Here's how the part is built. I have some questions about the finished solid (model axes, mm). Face numbers are marked on the shaded views. A direction names the side the tool comes from. Coordinates: 2 decimals unless noted, no trailing zeros. Write each loop counter-clockwise with the first axis right and the second up, starting at its lowest first coordinate (ties: lowest second). Pieces come first, ordered by that corner, then holes. Notation, with made-up numbers: (15.5, 24.25) -> (23.5, 24.25) arc R10 ccw to (23.5, 31.25) -> close; hole circle Ø9 at (54, -17). An arc over 180 degrees is marked (long way). Put each result on its own line as item: value. Start each with the question number.
Item 1: On a 3-axis mill with a long thin cutter (end or side, diameter ignored), from which of +Z, -Z, +X, -X, +Y, -Y can I reach the whole of each face in a straight line? I mean the marked faces 5, 6, 7, 8 and 9. Say none if no direction works.
Item 2: I want a section at C-C, the plane z = 15. State how many separate pieces and enclosed holes the cut face has, then the cut area to 3 significant figures.
Item 3: For pin 1 (1.5 mm diameter, centred on x = 102.5, z = 7, fed in from +Y); pin 2 (4 mm diameter, centred on x = 70, z = 23, fed in from -Y); pin 3 (13 mm diameter, centred on x = 114.5, z = 18, fed in from +Y); pin 4 (3 mm diameter, centred on y = -4.5, z = 17, fed in from -X), each with a flat end and sliding along its axis, tell me the tip position at first contact or that it passes through.
Item 4: If we mould it in two halves opening along Z, with no side actions, what happens to the marked faces 1, 2, 3 and 4? For each: released by +Z, released by -Z, zero draft, split by the parting line, or undercut.
Item 5: I want a section at B-B, the plane x = 21.5. List the corners of the cut face in (y, z) for me, then the cut area to 3 significant figures.
Item 6: I need wall thicknesses on line 1 (X direction, y = 16.05, z = 15); line 2 (Z direction, x = 70, y = 15.7); line 3 (Z direction, x = 78, y = 17.8). Which ranges of each line are inside material? Lowest first, please. Write a range as [from, to].
Item 7: I want a section at A-A, the plane y = 10.5. List the corners of the cut face in (x, z) for me.
Autodesk Inventor part; units mm, degrees
ref_plane "YZ Plane" through (0, 0, 0) normal (1, 0, 0) x (0, 1, 0)
ref_plane "XZ Plane" through (0, 0, 0) normal (0, 1, 0) x (-1, 0, 0)
ref_plane "XY Plane" through (0, 0, 0) normal (0, 0, 1) x (1, 0, 0)
sketch "Sketch1" plane through (0, 0, 0) normal (0, 0, 1) x (1, 0, 0)
  line L0 (5, 0) -> (50, 0)
  line L1 (50, 0) -> (50, 18)
  line L2 (52, 20) -> (88, 20)
  line L3 (90, 18) -> (90, 0)
  line L4 (105, 0) -> (135, 0)
  line L5 (140, -5) -> (140, -10)
  line L6 (140, -10) -> (87, -10)
  line L7 (53, -10) -> (0, -10)
  line L8 (0, -10) -> (0, -5)
  line L9 (57, 15) -> (83, 15)
  line L10 (55, 13) -> (55, -8)
  line L11 (85, -8) -> (85, 13)
  arc A0 (52, 20) -> (50, 18) centre (52, 18) ccw
  arc A1 (90, 18) -> (88, 20) centre (88, 18) ccw
  line L12 (50, 9) -> (35, 0)
  line L13 (90, 0) -> (90, 9)
  line L14 (90, 9) -> (105, 0)
  arc A2 (57, 15) -> (55, 13) centre (57, 13) ccw
  arc A3 (85, 13) -> (83, 15) centre (83, 13) ccw
  arc A4 (53, -10) -> (55, -8) centre (53, -8) ccw
  arc A5 (85, -8) -> (87, -10) centre (87, -8) ccw
  line L15 (5, 0) -> (0, -5)
  line L16 (135, 0) -> (140, -5)
  point P0 (0, 0)
  point P1 (50, 20)
  point P2 (90, 20)
  point P3 (140, 0)
  point P4 (140, 0)
  point P5 (0, 0)
  point P6 (140, 0)
  dimension "d0" = 50
  dimension "d1" = 20
  dimension "d2" = 40
  dimension "d3" = 50
  dimension "d4" = 10
  dimension "d7" = 10
  dimension "d8" = 5
  dimension "d9" = 2
  dimension "d10" = 15
  dimension "d11" = 9
  dimension "d12" = 15
  dimension "d13" = 2
  dimension "d14" = 30
  dimension "d15" = 2
  dimension "d18" = 5
  dimension "d19" = 5
  dimension "d20" = 5
  dimension "d21" = 5
extrude "Extrusion1" add sketch "Sketch1" along normal blind 30
sketch "Sketch2" plane through (105, 0, 0) normal (0, 1, 0) x (1, 0, 0)
  circle A0 centre (15, -15) radius 6.5
  line L0 (30, 0) -> (0, 0)
  line L1 (0, 0) -> (0, -30)
  circle A1 centre (-84.9999, -15) radius 6.5
  line L2 (-100, 0) -> (-100, -30)
  line L3 (-70, 0) -> (-100, 0)
  point P0 (-105, 0)
  point P1 (0, -15)
  dimension "d24" = 13
  dimension "d25" = 15
  dimension "d26" = 15
  dimension "d27" = 13
  dimension "d28" = 15
  dimension "d29" = 15
extrude "Extrusion2" cut sketch "Sketch2" against normal blind 30
sketch "Sketch3" plane through (0, 0, 30) normal (0, 0, 1) x (1, 0, 0)
  point P0 (0, 0)
sketch "Sketch4" plane through (52, 20, 0) normal (0, 1, 0) x (1, 0, 0)
  circle A0 centre (18, -15) radius 11.75
  line L0 (38, 0) -> (38, -30)
  line L1 (36, 0) -> (0, 0)
  circle A1 centre (18, -7) radius 1.6
  circle A2 centre (10, -15) radius 1.6
  circle A3 centre (18, -23) radius 1.6
  circle A4 centre (26, -15) radius 1.6
  point P0 (-52, 0)
  dimension "d32" = 23.5
  dimension "d33" = 20
  dimension "d34" = 15
  dimension "d35" = 3.2
  dimension "d36" = 8
  dimension "d39" = 360
extrude "Extrusion3" cut sketch "Sketch4" against normal blind 1.5
extrude "Extrusion4" cut sketch "Sketch4" against normal blind 30 contours A1 | A2 | A3 | A4
fillet "Fillet1" radius 2 18 edges at (50.5858, 19.4142, 0) (50, 13.5, 0) (89.4142, 19.4142, 0) (90, 13.5, 0) (70, 20, 0) (50.5858, 19.4142, 30) (50, 13.5, 30) (89.4142, 19.4142, 30) (90, 13.5, 30) (70, 20, 30) (97.5, 4.5, 30) (120, 0, 30) (97.5, 4.5, 0) (120, 0, 0) (42.5, 4.5, 30) (20, 0, 30) (20, 0, 0) (42.5, 4.5, 0)
chamfer "Chamfer1" distance 0.5 angle 45 1 edges at (58.25, 20, 15)
sketch "Sketch5" plane through (105, 0, 28) normal (0, 1, 0) x (1, 0, 0)
  point P0 (-105, 28)
equation "\"BendRadius\" = Thickness"
equation "\"BendReliefWidth\" = Thickness"
equation "\"BendReliefDepth\" = 0.5 * Thickness"
equation "\"CornerReliefSize\" = 4 * Thickness"
equation "\"MinimumRemnant\" = 2 * Thickness"
equation "\"TransitionRadius\" = BendRadius"
equation "\"JacobiRadiusSize\" = BendRadius"
equation "\"GapSize\" = Thickness"
properties part number "4_DOF_2"
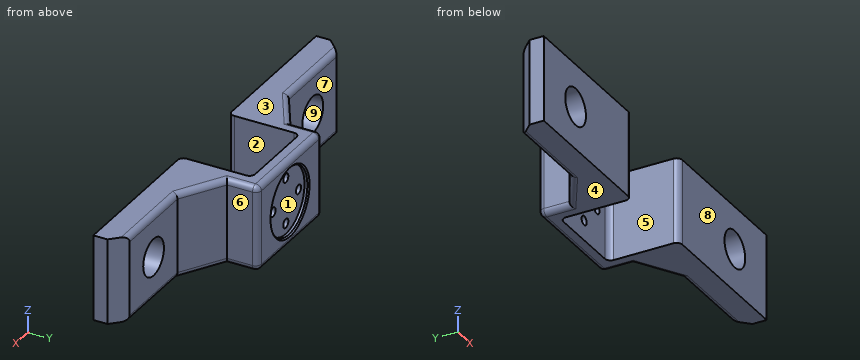
Calculated:
1. face 5: +Z, -Z, -Y
1. face 6: +Z, -Z, +X, +Y
1. face 7: +Z, -Z, -X, +Y
1. face 8: +Z, -Z, +X, -X, -Y
1. face 9: +Y, -Y
2. separate pieces: 5
2. enclosed holes: 0
2. area: 1,240 mm2
3. pin 1: stops at y = 1.95
3. pin 2: stops at y = 15
3. pin 3: stops at y = 0
3. pin 4: stops at x = 0
4. face 1: undercut
4. face 2: zero draft
4. face 3: released by +Z
4. face 4: released by -Z
5. outline: (-10, 0) -> (-2, 0) arc R2 ccw to (0, 2) -> (0, 8.68) -> (-10, 8.68) -> close; (-10, 21.32) -> (0, 21.32) -> (0, 28) arc R2 ccw to (-2, 30) -> (-10, 30) -> close
5. area: 172 mm2
6. line 1: x = [50, 60.4], [63.6, 76.4], [79.6, 90]
6. line 2: z = [0, 5.4], [8.6, 21.4], [24.6, 30]
6. line 3: z = [0, 13.4], [16.6, 30]
7. outline: (50, 2) arc R2 ccw to (52, 0) -> (55, 0) -> (55, 30) -> (52, 30) arc R2 ccw to (50, 28) -> close; (85, 0) -> (88, 0) arc R2 ccw to (90, 2) -> (90, 28) arc R2 ccw to (88, 30) -> (85, 30) -> close
